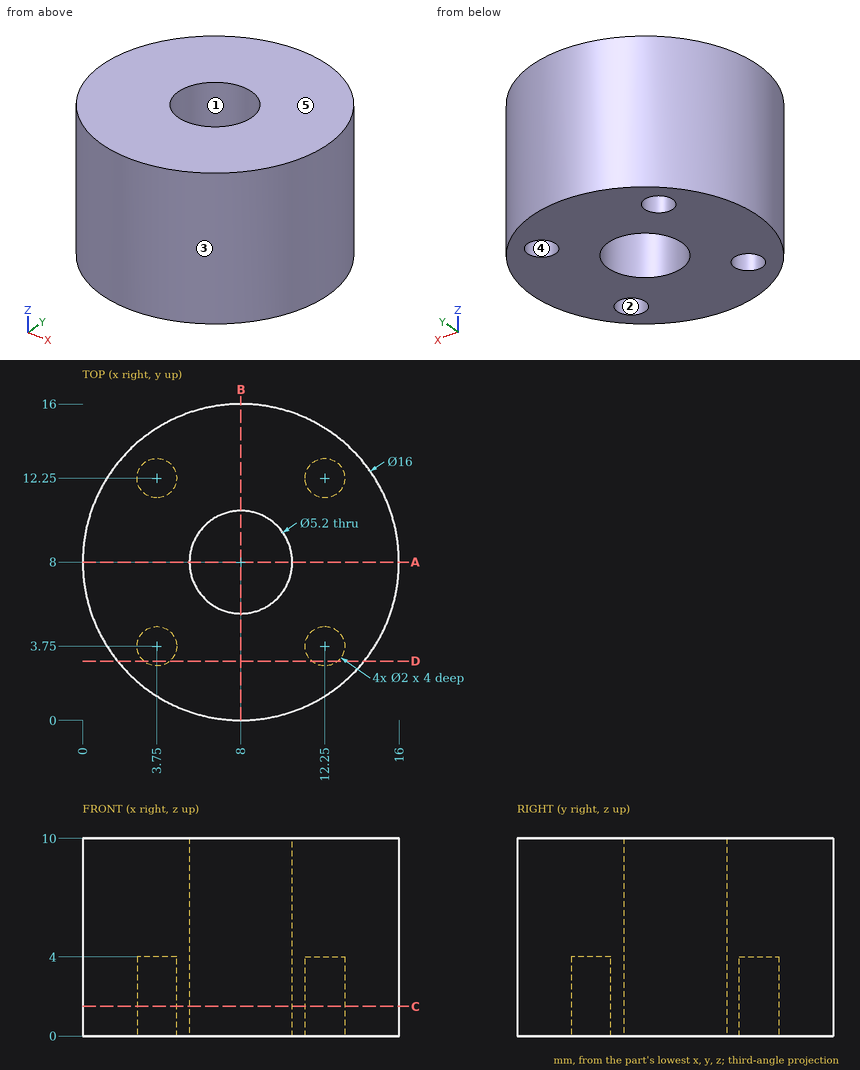
Drawing for the job (mm, zero at the part's lowest x, y, z). A direction names the side the tool comes from. Coordinates: 2 decimals unless noted, no trailing zeros. Order: outer loops, then holes, each group sorted by start corner. A loop starts at its lowest first (then second) coordinate and runs counter-clockwise, first axis right, second up.
Item 1: Two-plate mould, pull along X, no slides. Class the marked faces 3, 4 and 5: +X half, -X half, draft (parallel to the pull), parting line (faces both ways), or undercut.
Check sheet entries:
face 3: parting line
face 4: undercut
face 5: draft
Item 2: 3-axis set-ups, long thin cutter, end or side, ignore diameter. For the marked faces 1 and 2: which of +Z, -Z, +X, -X, +Y, -Y reach the whole face in a straight line?
Check sheet entries:
face 1: +Z, -Z
face 2: -Z
Item 3: Band-saw the part on D-D on y = 3. List the corners of the cut face in (x, z) (3 decimals), plus the area to 3 significant figures.
Check sheet entries:
outline: (1.755, 0) - (3.089, 0) - (3.089, 4) - (4.411, 4) - (4.411, 0) - (11.589, 0) - (11.589, 4) - (12.911, 4) - (12.911, 0) - (14.245, 0) - (14.245, 10) - (1.755, 10) - close
area: 114 mm2
Item 4: Drill centre lines: L1, parallel to Y at x = 8, z = 5.5; L2, parallel to Y at x = 12.25, z = 1.8. Where is each one in solid material? Low to high.
Check sheet entries:
L1: y = 0 to 5.4, 10.6 to 16
L2: y = 1.22 to 2.75, 4.75 to 11.25, 13.25 to 14.78
Item 5: Band-saw the part on C-C on z = 1.5. List the corners of the cut face in (x, y), plus the area to 3 significant figures.
Check sheet entries:
outline: circle Ø16 at (8, 8); hole circle Ø2 at (3.75, 3.75); hole circle Ø2 at (3.75, 12.25); hole circle Ø5.2 at (8, 8); hole circle Ø2 at (12.25, 3.75); hole circle Ø2 at (12.25, 12.25)
area: 167 mm2
Item 6: Band-saw the part on A-A on y = 8. List the corners of the cut face in (x, z), plus the area to 3 significant figures.
Check sheet entries:
outline: (0, 0) - (5.4, 0) - (5.4, 10) - (0, 10) - close; (10.6, 0) - (16, 0) - (16, 10) - (10.6, 10) - close
area: 108 mm2
Item 7: Pin check, flat tips, straight feed: pin 1 Ø1.8 at (x, y) = (3.75, 12.25) entering from -Z; pin 2 Ø1 at (y, z) = (14.5, 2.5) entering from +X; pin 3 Ø3 at (y, z) = (11.5, 4.5) entering from +X. Stop position of each tip, or through.
Check sheet entries:
pin 1: stops at z = 4
pin 2: stops at x = 13.29
pin 3: stops at x = 15.75
